```python
from build123d import *

# Parameters (mm, degrees)
CUT_EXTRUDE_1_DEPTH      = 67.708320321
PATTERN_CIRCULAR_1_COUNT = 3


with BuildPart() as part:
    # 草图1 → 旋转1 (revolve)
    with BuildSketch(Plane.XY, mode=Mode.PRIVATE) as revolve_1_sk:
        Polygon((10, 26), (10, 6), (37, 6), (43, 12), (45, 12), (45, 0), (3, 0), (3, 23), (5.5, 23), (5.5, 26), align=None)
    revolve(revolve_1_sk.sketch.rotate(Axis((0, 83.728815318, 0), (0, -1, 0)), 90), axis=Axis((0, 83.728815318, 0), (0, -1, 0)))

    # 草图2 → 切除-拉伸1 (cut, symmetric)
    with BuildSketch(Plane(origin=(0, 6, 0), x_dir=(1, 0, 0), z_dir=(0, 1, 0))):
        with BuildLine():
            Line((-15.696380071, 22), (39.255572853, 22))
            ThreePointArc((39.255572853, 22), (39.795996859, 21.006633096), (40.311288741, 20))
            Line((40.311288741, 20), (-15.696380071, 20))
            ThreePointArc((-15.696380071, 20), (-28.618996361, 21), (-15.696380071, 22))
        make_face()
    cut_extrude_1 = extrude(amount=CUT_EXTRUDE_1_DEPTH, both=True, mode=Mode.SUBTRACT)

    # 阵列(圆周)1: 切除-拉伸1 ×3 about axis
    pattern_circular_1_axis = Axis((0, 0, 0), (0, 1, 0))
    for i in range(1, PATTERN_CIRCULAR_1_COUNT):
        add(cut_extrude_1.rotate(pattern_circular_1_axis, i * 360 / PATTERN_CIRCULAR_1_COUNT), mode=Mode.SUBTRACT)


solid = part.part
```
Geometry: final body of the model. Coordinates: model frame, mm. A direction names the side the tool comes from. Coordinates: 2 decimals unless noted, no trailing zeros. Order: outer loops, then holes, each group sorted by start corner. A loop starts at its lowest first (then second) coordinate and runs counter-clockwise, first axis right, second up. Notation, with made-up numbers: (48.5, 86.25) -> (65.5, 86.25) arc R17 cw to (65.5, 111.25) -> close; hole circle Ø9 at (53, -11.5). An arc over 180 degrees is marked (long way). Answer in a Markdown table with one row per item.
Item 1: Section A-A on y = 10.75. Output: boundary loops of the cut face in (x, z), plus the area to 3 significant figures.
Return value:
| item | result |
|---|---|
| outline | (-38.68, -23) -> (-36.79, -19.73) arc R41.75 cw to (-1, 41.74) -> (-2.84, 44.91) arc R45 ccw to start; (-37.48, -24.91) arc R45 ccw to (39.26, -22) -> (35.48, -22) arc R41.75 cw to (-35.64, -21.74) -> close; circle Ø20 at (0, 0); (-0.58, 45) -> (1.31, 41.73) arc R41.75 cw to (36.65, -20) -> (40.31, -20) arc R45 ccw to start; hole circle Ø6 at (0, 0) |
| area | 1,150 mm² |
Item 2: Section D-D on x = 8.5. State how many separate pieces and enclosed holes the cut face has, plus the area to 3 significant figures.
Return value:
| item | result |
|---|---|
| separate pieces | 3 |
| enclosed holes | 0 |
| area | 766 mm² |
Item 3: Draft query along Z for faces 1 (the flat face through (-38, 12, 21)), 2 (the cylindrical face through (-39.491, 5.916, 21.574)), 3 (the conical face through (-31.49, 6.38, 20.14)). Return one class per face: released by +Z, released by -Z, zero draft, split by the parting line, or undercut.
Return value:
| item | result |
|---|---|
| face 1 | zero draft |
| face 2 | split by the parting line |
| face 3 | undercut |
Item 4: Section B-B on z = 0. Output: boundary loops of the cut face in (x, y).
Return value:
| item | result |
|---|---|
| outline | (-45, 0) -> (-25.4, 0) -> (-25.4, 6) -> (-37, 6) -> (-43, 12) -> (-45, 12) -> close; (-23.09, 0) -> (-3, 0) -> (-3, 23) -> (-5.5, 23) -> (-5.5, 26) -> (-10, 26) -> (-10, 6) -> (-23.09, 6) -> close; (3, 0) -> (23.09, 0) -> (23.09, 6) -> (10, 6) -> (10, 26) -> (5.5, 26) -> (5.5, 23) -> (3, 23) -> close; (25.4, 0) -> (45, 0) -> (45, 12) -> (43, 12) -> (37, 6) -> (25.4, 6) -> close |
Item 5: Access query for faces 4 (the flat face through (2.4, 23, -2.4)), 5 (the flat face through (36, 12, 25)), 6 (the flat face through (11, 3, -22)), 7 (the flat face through (-26.782, 3.417, -6.387)). Directions: +Z, -Z, +X, -X, +Y, -Y. A direction counts if a zero-diameter tool reaches every point of the face in a straight line with its end or side. Return the directions, or none.
Return value:
| item | result |
|---|---|
| face 4 | +Y |
| face 5 | +Z, +X, +Y |
| face 6 | +X, +Y, -Y |
| face 7 | +Y, -Y |
Item 6: Ray query, L1, parallel to X at y = 25.45, z = 0; L2, parallel to Y at x = -4, z = -18.5; L3, parallel to Z at x = 0.5, y = 10. Return the intervals inside material, ascending.
Return value:
| item | result |
|---|---|
| L1 | x = -10 to -5.5, 5.5 to 10 |
| L2 | y = 0 to 6 |
| L3 | z = -45 to -41, -9.99 to -2.96, 2.96 to 9.99, 43.13 to 45 |
Item 7: Contact query for flat-ended pins moving along their axis: P1, Ø1, axis at x = 10, y = 8.5, coming from the -Z side; P2, Ø3, axis at x = 23, y = 9.5, coming from the -Z side; P3, Ø4.5, axis at x = 8.5, z = -31, coming from the +Y side; P4, Ø10.5, axis at x = 29.25, z = -8.66, coming from the -Y side. Output: stop coordinate, or through.
Return value:
| item | result |
|---|---|
| P1 | stops at z = -43.99 |
| P2 | stops at z = -39.53 |
| P3 | stops at y = 6 |
| P4 | passes through |
Item 8: Section C-C on y = 17. Output: boundary loops of the cut face in (x, z), plus the area to 3 significant figures.
Return value:
| item | result |
|---|---|
| outline | circle Ø20 at (0, 0); hole circle Ø6 at (0, 0) |
| area | 286 mm² |
